```python
from build123d import *

# Parameters (mm, degrees)
PAD_DEPTH    = 53
SKETCH001_W  = 2
SKETCH001_H  = 4.6
POCKET_DEPTH = 0.6


with BuildPart() as part:
    # Sketch → Pad (new body)
    with BuildSketch(Plane.YZ):
        with BuildLine():
            ThreePointArc((-14.15, 2.8), (-16.95, 0), (-14.15, -2.8))
            Line((-14.15, -2.8), (14.15, -2.8))
            ThreePointArc((14.15, -2.8), (16.95, 0), (14.15, 2.8))
            Line((-14.15, 2.8), (14.15, 2.8))
        make_face()
    extrude(amount=PAD_DEPTH)

    # Sketch001 (on DatumPlane) → Pocket (cut)
    with BuildSketch(Plane(origin=(0, 0, 0), x_dir=(0, 1, 0), z_dir=(-1, 0, 0))):
        with Locations((12.95, 0)):
            Rectangle(SKETCH001_W, SKETCH001_H)
        with Locations((9.75, 0)):
            Rectangle(SKETCH001_W, SKETCH001_H)
        with Locations((6.55, 0)):
            Rectangle(SKETCH001_W, SKETCH001_H)
    extrude(amount=-POCKET_DEPTH, mode=Mode.SUBTRACT)


solid = part.part
```
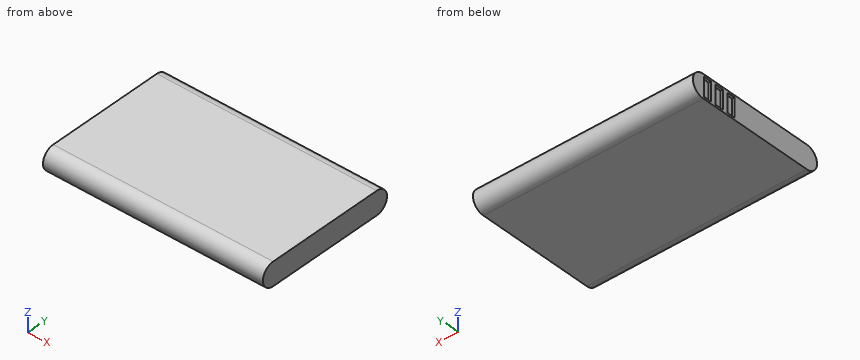
Can you work these out from the model? Positions are in its coordinate system, mm. Round coordinates to 2 decimals unless told otherwise and drop trailing zeros. Order: outer loops, then holes, each group sorted by start corner. A loop starts at its lowest first (then second) coordinate and runs counter-clockwise, first axis right, second up.
(1) If we section it at A-A (x = 11): Please give me the cut outline in (y, z), plus the area to 3 significant figures.
Results are:
outline: (-14.15, -2.8) - (14.15, -2.8) arc R2.8 ccw to (14.15, 2.8) - (-14.15, 2.8) arc R2.8 ccw to start
area: 183 mm2
(2) If I drill on L1, parallel to X at y = 7, z = 0.9; L2, parallel to Y at x = 26.5, z = -0.15; L3, parallel to Y at x = 8.5, z = 2, over which ranges is the centre line in solid material (lowest first)?
Results are:
L1: x = 0.6 to 53
L2: y = -16.95 to 16.95
L3: y = -16.11 to 16.11
(3) I'm going to push flat-ended pins straight in: pin 1 (0.7 mm diameter, centred on x = 0.5, z = -1, fed in from +Y); pin 2 (1.5 mm diameter, centred on x = 35, z = -2, fed in from +Y); pin 3 (0.5 mm diameter, centred on x = 0.5, z = 1, fed in from +Y). Where does each tip first touch, or does it pass through?
Results are:
pin 1: stops at y = 16.87
pin 2: stops at y = 16.66
pin 3: stops at y = 16.85
